Drawing for the job (mm, zero at the part's lowest x, y, z). A direction names the side the tool comes from. Coordinates: 2 decimals unless noted, no trailing zeros. Write each loop counter-clockwise with the first axis right and the second up, starting at its lowest first coordinate (ties: lowest second). Pieces come first, ordered by that corner, then holes. Notation, with made-up numbers: M -30,1.5 L 10,1.5 A21 cw 10,33.5 Z; hole C 38.5,71 d9. An arc over 180 degrees is marked long. Put each result on its own line as item: value. Start each with the question number.
Q1. Cut at B-B (x = 12.5). Write the cut outline in (y, z), then the cut area to 3 significant figures.
Q2. Cut at A-A (z = 1.5). Write the cut outline in (x, y), then the cut area to 3 significant figures.
Q3. Drill centre lines: line 1 along Y through (x, z) = (10.5, 12.5); line 2 along X through (y, z) = (12.75, 3.25); line 3 along Y through (x, z) = (8.5, 4.25). Where is each one in solid material? Low to high.
Q4. Cut at D-D (x = 7). Write the cut outline in (y, z), then the cut area to 3 significant figures.
Q5. Which spindle directions (+Z, -Z, +X, -X, +Y, -Y) get a long thin tool onto all of the face, cutting with end or side? Do the marked faces 1, 2 and 3. Say none if no direction does.
Q6. Cut at C-C (y = 10.5). Write the cut outline in (x, z), then the cut area to 3 significant figures.
Q7. Drop flat-ended pins along their axis: pin 1 (4 mm diameter, centred on y = 8.5, z = 7, fed in from -X); pin 2 (4 mm diameter, centred on x = 6, z = 3.5, fed in from +Y); pin 3 (4 mm diameter, centred on x = 8, y = 3.5, fed in from -Z); pin 4 (5.5 mm diameter, centred on y = 13.5, z = 3.5, fed in from -X). Give the stop position or say it passes through.
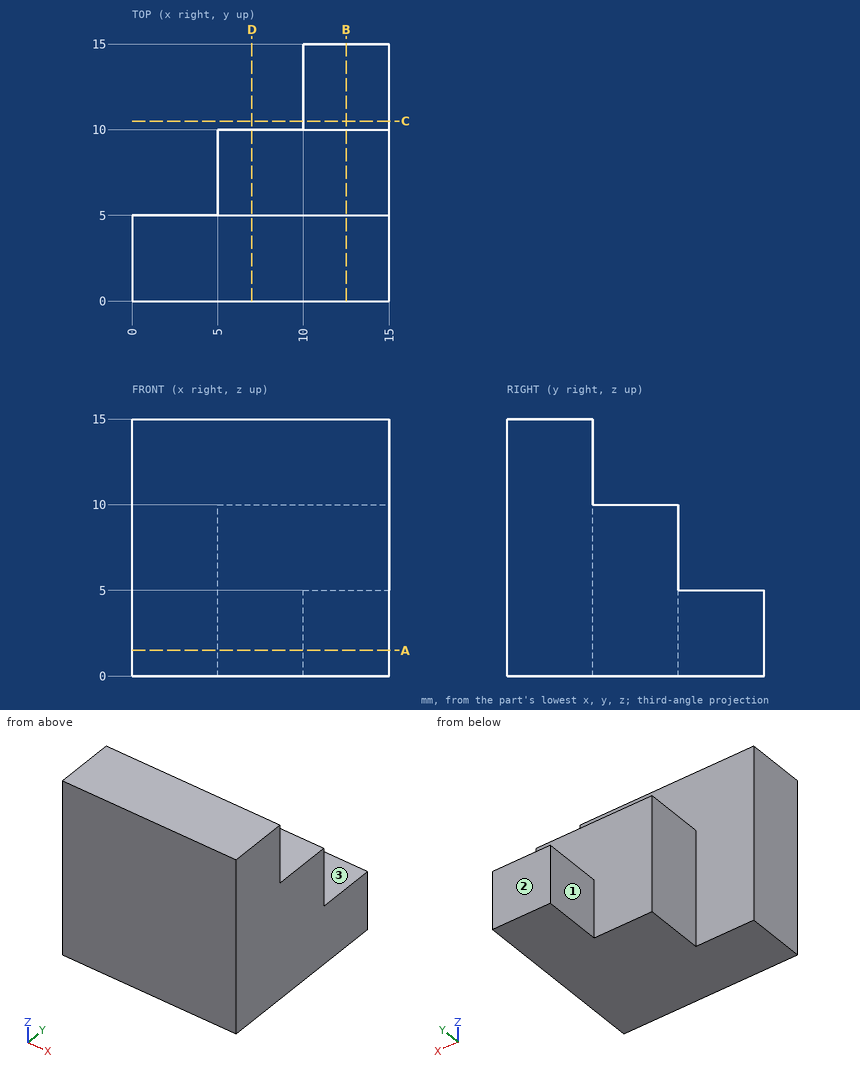
Computed values:
1. outline: M 0,0 L 15,0 L 15,5 L 10,5 L 10,10 L 5,10 L 5,15 L 0,15 Z
1. area: 150 mm2
2. outline: M 0,0 L 15,0 L 15,15 L 10,15 L 10,10 L 5,10 L 5,5 L 0,5 Z
2. area: 150 mm2
3. line 1: 0 to 5
3. line 2: 10 to 15
3. line 3: 0 to 10
4. outline: M 0,0 L 10,0 L 10,10 L 5,10 L 5,15 L 0,15 Z
4. area: 125 mm2
5. face 1: +Z, -Z, -X, +Y
5. face 2: +Z, -Z, +X, -X, +Y
5. face 3: +Z, +X, -X, +Y
6. outline: M 10,0 L 15,0 L 15,5 L 10,5 Z
6. area: 25.0 mm2
7. pin 1: x = 5
7. pin 2: y = 10
7. pin 3: z = 0
7. pin 4: x = 10
